from build123d import *

# Parameters (mm, degrees)
F1_DEPTH = 10
F2_R     = 2.1
F3_DEPTH = 5.001
F5_ANGLE = 90


with BuildPart() as f1:
    # F0 (on Right) → F1 (new body)
    with BuildSketch(Plane.YZ):
        Polygon((-10, 0), (0, 0), (0, 165), (-5, 165), (-5, 175), (-10, 175), align=None)
    extrude(amount=F1_DEPTH)

    # F2 (on face) → F3 (cut, through all)
    with BuildSketch(Plane(origin=(0, -5, 0), x_dir=(-1, 0, 0), z_dir=(0, 1, 0))):
        with Locations((-5, 170)):
            Circle(F2_R)
    extrude(amount=-F3_DEPTH, mode=Mode.SUBTRACT)

    # F4: F1 across plane


with BuildPart() as f1_1:
    add(f1.part)
    add(f1.part.mirror(Plane.XY))


with BuildPart() as f1_2:
    # F5: moved
    add(f1_1.part.rotate(Axis((0, -5, 0), (0, 1, 0)), F5_ANGLE))


solid = f1_2.part
For this review, take the finished solid that the model builds, in its own axes (mm). A direction names the side the tool comes from. Give positions to 0.01 mm unless a question says otherwise; leave off trailing zeros. Order: outer loops, then holes, each group sorted by start corner. A loop starts at its lowest first (then second) coordinate and runs counter-clockwise, first axis right, second up. Notation, with made-up numbers: (84.25, 49.5) -> (123.25, 49.5) arc R30 ccw to (123.25, 80.5) -> close; hole circle Ø8 at (36, -22.75). An arc over 180 degrees is marked (long way). Write item = value, one per line.
1) Insertion check: pin 1 (1.5 mm diameter, centred on y = -3.5, z = -4, fed in from -X); pin 2 (1.5 mm diameter, centred on y = -3.5, z = -7, fed in from +X); pin 3 (5 mm diameter, centred on x = 170, z = -5, fed in from +Y). Each pin has a flat end and moves straight along its axis. Give the tip position at first contact, or say it passes through.
Findings:
pin_1 = -165
pin_2 = 165
pin_3 = -5
2) We need section A-A, the plane z = -5. Give the boundary of the cut face in (x, y).
Findings:
outline = (-175, -10) -> (-172.1, -10) -> (-172.1, -5) -> (-175, -5) -> close; (-167.9, -10) -> (167.9, -10) -> (167.9, -5) -> (165, -5) -> (165, 0) -> (-165, 0) -> (-165, -5) -> (-167.9, -5) -> close; (172.1, -10) -> (175, -10) -> (175, -5) -> (172.1, -5) -> close
3) To check wall thickness, follow L1, parallel to X at y = -6.1, z = -5; L2, parallel to Z at x = 170, y = -6.55; L3, parallel to X at y = -1.25, z = -3. State the ranges of each line that lie inside material, in increasing order. Write a range as from..to.
Findings:
L1 = -175..-172.1, -167.9..167.9, 172.1..175
L2 = -10..-7.1, -2.9..0
L3 = -165..165
4) We need section B-B, the plane y = -2.5. Give the boundary of the cut face in (x, z), and give its area (3 significant figures).
Findings:
outline = (-165, -10) -> (165, -10) -> (165, 0) -> (-165, 0) -> close
area = 3,300 mm^2
5) For faces 1 (the face through (167.7, -5, -4.9)), 2 (the face through (-2, -5, -10)), 3 (the face through (-167.7, -5, -4.9)), list the 3-axis set-ups (+Z, -Z, +X, -X, +Y, -Y) from which the entire face can be reached by the end or side of a thin tool; tool diameter is ignored.
Findings:
face_1 = +Z, -Z, +X, +Y
face_2 = -Z, +X, -X, +Y, -Y
face_3 = +Z, -Z, -X, +Y
